```python
from build123d import *

# Parameters (mm, degrees)
SKETCH_1_R              = 14
SKETCH_1_R_2            = 11.4
RING_DEPTH              = 5
STICK_DEPTH             = 5
FILLET_1_R              = 5
CORRECTION_HOLE_1_DEPTH = 161.68914089
CUT_EXTRUDE_1_REACH     = 163.087
FILLET_2_R              = 4
SKETCH_10_R             = 10
EXTRUDE_2_DEPTH         = 30
SKETCH_11_R             = 4.25
CUT_EXTRUDE_3_DEPTH     = 30
SKETCH_12_W             = 14.282856858
SKETCH_12_H             = 1
CUT_EXTRUDE_4_DEPTH     = 5
SKETCH_13_W             = 14.282856858
SKETCH_13_H             = 1
CUT_EXTRUDE_6_DEPTH     = 5


with BuildPart() as part:
    # Эскиз1 → ring (new body)
    with BuildSketch(Plane(origin=(0, 0, 0), x_dir=(1, 0, 0), z_dir=(0, 1, 0))):
        with Locations(Location((0, 0, 0), (0, 0, 270))):
            Circle(SKETCH_1_R)
        with Locations(Location((0, 0, 0), (0, 0, 270))):
            Circle(SKETCH_1_R_2, mode=Mode.SUBTRACT)
    extrude(amount=RING_DEPTH)

    # Эскиз2 → stick (add)
    with BuildSketch(Plane(origin=(0, 0, 0), x_dir=(1, 0, 0), z_dir=(0, 1, 0))):
        with BuildLine():
            Line((-10.781929326, 4), (-160, 4))
            Line((-160, 4), (-160, -4))
            Line((-160, -4), (-10.781929326, -4))
            ThreePointArc((-10.781929326, -4), (-11.5, 0), (-10.781929326, 4))
        make_face()
    extrude(amount=STICK_DEPTH)

    # Скругление1
    fillet_1_edges = [part.edges().sort_by_distance(p)[0] for p in [
        (-13.416407865, 2.5, 4),
        (-13.416407865, 2.5, -4),
    ]]
    fillet(fillet_1_edges, radius=FILLET_1_R)

    # Эскиз5 → correction hole 1 (cut, through all)
    with BuildSketch(Plane.XZ):
        Polygon((-75.4, -4), (-75.4, -1.5), (0, -1.5), (0, -1.7), (-75, -1.7), (-75, -4), align=None)
    extrude(amount=-CORRECTION_HOLE_1_DEPTH, mode=Mode.SUBTRACT)

    # Эскиз9 → Вытянуть1 (cut, up to next)
    with BuildSketch(Plane.XY.offset(4), mode=Mode.PRIVATE) as cut_extrude_1_sk1:
        Polygon((-142, 5), (-142, 4.1), (-143, 3.1), (-156, 3.1), (-156, 1.9), (-141.8, 1.9), (-140.8, 2.9), (-140.8, 5), align=None)
    cut_extrude_1_tool1 = extrude(cut_extrude_1_sk1.sketch, amount=-CUT_EXTRUDE_1_REACH, mode=Mode.PRIVATE) & part.part
    add(cut_extrude_1_tool1.solids().sort_by_distance((-147.651462, 2.701462, 4))[0], mode=Mode.SUBTRACT)

    # Скругление2
    fillet_2_edges = [part.edges().sort_by_distance(p)[0] for p in [
        (-156, 2.5, -4),
        (-156, 2.5, 4),
    ]]
    fillet(fillet_2_edges, radius=FILLET_2_R - 0.0001)  # a hair under: the kernel refuses the full size

    # Эскиз10 → Вытянуть2 (add)
    with BuildSketch(Plane(origin=(0, 5, 0), x_dir=(1, 0, 0), z_dir=(0, 1, 0))):
        with Locations(Location((-100, 0, 0), (0, 0, 270))):
            Circle(SKETCH_10_R)
    extrude(amount=-EXTRUDE_2_DEPTH)

    # Эскиз11 → Вытянуть3 (cut)
    with BuildSketch(Plane.XZ.offset(25)):
        with Locations(Location((-100, 0, 0), (0, 0, 270))):
            Circle(SKETCH_11_R)
    extrude(amount=-CUT_EXTRUDE_3_DEPTH, mode=Mode.SUBTRACT)

    # Эскиз12 → Вытянуть4 (cut)
    with BuildSketch(Plane.XZ.offset(25)):
        with Locations((-100, -7.5)):
            Rectangle(SKETCH_12_W, SKETCH_12_H)
    extrude(amount=-CUT_EXTRUDE_4_DEPTH, mode=Mode.SUBTRACT)

    # Эскиз13 → Вытянуть6 (cut)
    with BuildSketch(Plane(origin=(0, 5, 0), x_dir=(1, 0, 0), z_dir=(0, 1, 0))):
        with Locations((-100, 7.5)):
            Rectangle(SKETCH_13_W, SKETCH_13_H)
    extrude(amount=-CUT_EXTRUDE_6_DEPTH, mode=Mode.SUBTRACT)


solid = part.part
```
Check sheet for the modelled part. Datum: model origin and axes. Units: mm. A direction names the side the tool comes from. Round coordinates to 2 decimals unless told otherwise and drop trailing zeros. Order: outer loops, then holes, each group sorted by start corner. A loop starts at its lowest first (then second) coordinate and runs counter-clockwise, first axis right, second up. Notation, with made-up numbers: (-37, 56.5) -> (-30, 56.5) arc R19 cw to (-30, 87.5) -> close; hole circle Ø5 at (-6, -8). An arc over 180 degrees is marked (long way). One line per item, written item: value. Start each with the question number.
Q1. Cross-section at A-A (x = -100). Record the boundary of the cut face in (y, z), and give its area (3 significant figures).
Q2. Cross-section at B-B (x = -69). Record the boundary of the cut face in (y, z).
Q3. Mould release check, pull along X, two halves, no side actions. Record for faces 1 (the face through (-135, 2, 4)), 2 (the face through (-43, 2, -1.7)): pulls with the +X half, pulls with the -X half, needs draft (parallel to the pull), parting line crosses it, or undercut.
Q4. Cross-section at D-D (z = 2). Record the boundary of the cut face in (x, y).
Q5. Gauge pin test, flat ends, axial feed: pin 1 Ø8 at (x, y) = (-48.5, -3.5) entering from -Z; pin 2 Ø3 at (y, z) = (3.5, -2.5) entering from +X; pin 3 Ø4 at (y, z) = (-8.5, -2) entering from -X. Record the tip position at first contact, or that the pin passes through.
Q6. Thickness scan on line 1 (X direction, y = 2.5, z = 4.5); line 2 (X direction, y = -18.75, z = -0.5); line 3 (Z direction, x = 0, y = 2.2). Record the ranges inside material, lowest first.
Q7. Cross-section at C-C (y = -6.75). Record the boundary of the cut face in (x, z).
Q8. Set-up check for faces 3 (the face through (-100, -23, -7)), 4 (the face through (-83, 2, -4)), 5 (the face through (-44, 2, -1.5)): record each of +Z, -Z, +X, -X, +Y, -Y from which the full face is reachable in a straight line by a thin tool's end or side.
Completed:
1. outline: (-25, -10) -> (5, -10) -> (5, -8) -> (0, -8) -> (0, -7) -> (5, -7) -> (5, -4.25) -> (-25, -4.25) -> (-25, -7) -> (-20, -7) -> (-20, -8) -> (-25, -8) -> close; (-25, 4.25) -> (5, 4.25) -> (5, 10) -> (-25, 10) -> close
1. area: 335 mm²
2. outline: (0, -4) -> (5, -4) -> (5, -1.7) -> (0, -1.7) -> close; (0, -1.5) -> (5, -1.5) -> (5, 4) -> (0, 4) -> close
3. face 1: needs draft
3. face 2: undercut
4. outline: (-160, 0) -> (-109.8, 0) -> (-109.8, -25) -> (-103.75, -25) -> (-103.75, 5) -> (-140.8, 5) -> (-140.8, 2.9) -> (-141.8, 1.9) -> (-156.54, 1.9) -> (-156.54, 3.1) -> (-143, 3.1) -> (-142, 4.1) -> (-142, 5) -> (-160, 5) -> close; (-96.25, -25) -> (-90.2, -25) -> (-90.2, 0) -> (-11.22, 0) -> (-11.22, 5) -> (-96.25, 5) -> close; (11.22, 0) -> (13.86, 0) -> (13.86, 5) -> (11.22, 5) -> close
5. pin 1: stops at z = -4
5. pin 2: stops at x = 13.96
5. pin 3: stops at x = -110
6. line 1: x = -108.93 to -91.07, -14.55 to -10.47, 10.47 to 13.26
6. line 2: x = -109.99 to -104.22, -95.78 to -90.01
6. line 3: z = -14 to -11.4, 11.4 to 14
7. outline: circle Ø20 at (-100, 0); hole circle Ø8.5 at (-100, 0)
8. face 3: +X, -X, -Y
8. face 4: -Z, +Y, -Y
8. face 5: +Y, -Y
